Input: dimensioned drawing with shaded views. Units: mm. Origin: part minimum x, y, z. A direction names the side the tool comes from. Coordinates: 2 decimals unless noted, no trailing zeros. Loops run counter-clockwise (first coordinate to the right, second up) from the corner with the lowest first, then second, coordinate; pieces in that order, holes last.
Item 1: Pull-direction query (X, two-part tool) for the marked faces 4, 5, 6 and 7; classes: +X half, -X half, draft (parallel to the pull), parting line (faces both ways), or undercut.
Item 2: Reachability of the marked faces 1, 2 and 3 from +Z, -Z, +X, -X, +Y, -Y: full face, straight path, thin tool, end or side. Return the list, or none.
Item 3: Line query: probe 1 along Z at (x, y) = (69, 32); probe 2 along Y at (x, z) = (23, 61); probe 3 along X at (y, z) = (44, 70.5). Output: solid intervals per line, ascending.
Item 4: Section query A-A, the plane x = 65. Return the cut outline in (y, z) (1 decimal), then the cut area to 3 significant figures.
Item 5: Section query D-D, the plane x = 46. Return the cut outline in (y, z).
Item 6: Section query B-B, the plane z = 102.5. Return the cut outline in (x, y).
Item 7: Pin query (flat end, axial travel): pin 1 Ø8 at (x, y) = (33, 39) entering from -Z; pin 2 Ø12 at (x, y) = (114, 36) entering from +Z; pin 3 Ø10 at (x, y) = (71.5, 14) entering from -Z. Return the tip coordinate at first contact, or that it passes through.
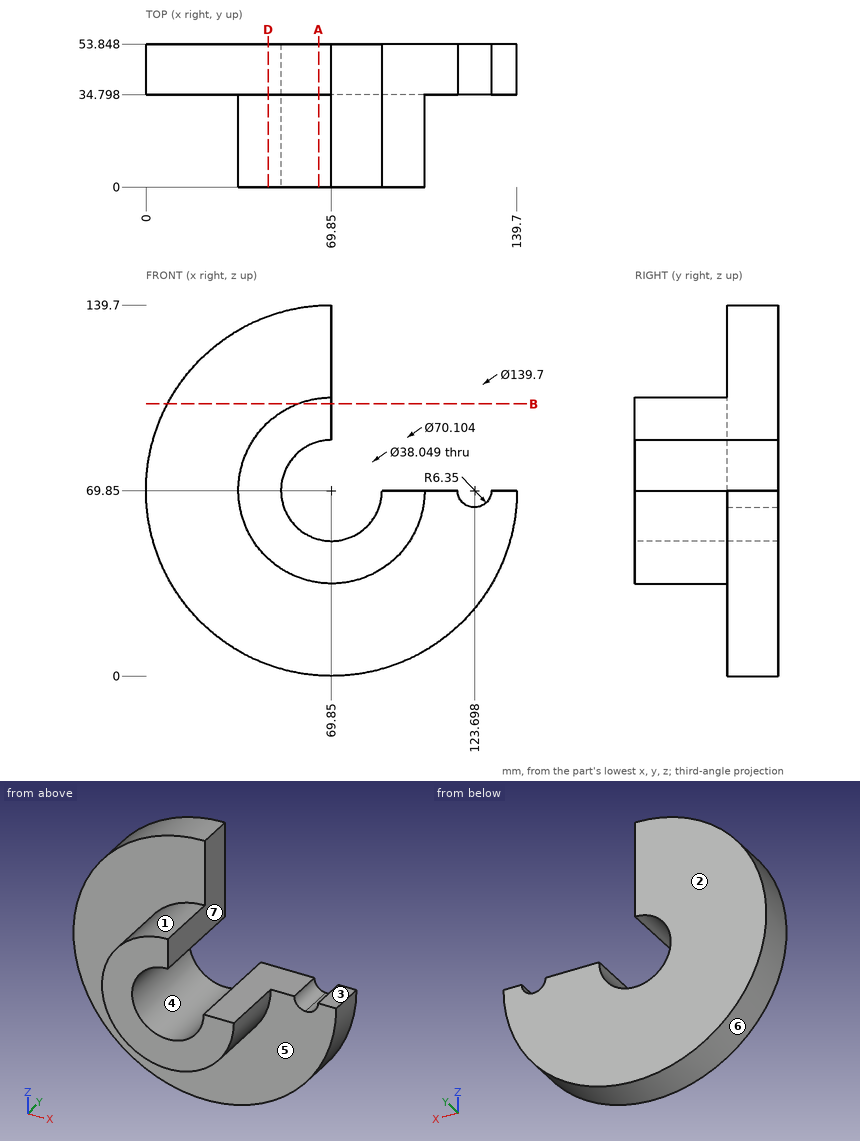
Verdict:
1. face 4: undercut
1. face 5: draft
1. face 6: parting line
1. face 7: +X half
2. face 1: -Y
2. face 2: +Z, -Z, +X, -X, +Y
2. face 3: +Z, +X, +Y, -Y
3. probe 1: z = 34.81 to 50.84, 88.86 to 104.89
3. probe 2: y = 34.8 to 53.85
3. probe 3: x = 0 to 50.84
4. outline: (0, 35.1) - (34.8, 35.1) - (34.8, 0.2) - (53.8, 0.2) - (53.8, 51.5) - (0, 51.5) - close; (0, 88.2) - (53.8, 88.2) - (53.8, 139.5) - (34.8, 139.5) - (34.8, 104.6) - (0, 104.6) - close
4. area: 3,090 mm2
5. outline: (0, 44.16) - (34.8, 44.16) - (34.8, 4.2) - (53.85, 4.2) - (53.85, 135.5) - (34.8, 135.5) - (34.8, 95.54) - (0, 95.54) - close
6. outline: (8.1, 34.8) - (57.1, 34.8) - (57.1, 0) - (69.85, 0) - (69.85, 53.85) - (8.1, 53.85) - close
7. pin 1: stops at z = 8.21
7. pin 2: stops at z = 69.85
7. pin 3: stops at z = 34.8
